from build123d import *

# Parameters (mm, degrees)
PAD_DEPTH       = 3
POCKET_DEPTH    = 2
SKETCH004_W     = 50
SKETCH004_H     = 84
SKETCH004_W_2   = 47.6
SKETCH004_H_2   = 81.6
POCKET001_DEPTH = 2
SKETCH005_R     = 3.5
SKETCH005_R_2   = 3
PAD001_DEPTH    = 6
SKETCH_R        = 1.8
POCKET002_DEPTH = 5


with BuildPart() as part:
    # Sketch002 → Pad (new body)
    with BuildSketch(Plane(origin=(0, 1, 0), x_dir=(-1, 0, 0), z_dir=(0, 1, 0))):
        Polygon((-44, -64), (2, -64), (2, 20), (-44, 20), (-48, 20), (-48, -64), align=None)
    extrude(amount=PAD_DEPTH)

    # Sketch003 → Pocket (cut)
    with BuildSketch(Plane(origin=(0, 1, 0), x_dir=(-1, 0, 0), z_dir=(0, 1, 0))):
        Polygon((-42, -62), (0, -62), (0, 18), (-42, 18), (-46, 18), (-46, -62), align=None)
    extrude(amount=POCKET_DEPTH, mode=Mode.SUBTRACT)

    # Sketch004 → Pocket001 (cut)
    with BuildSketch(Plane(origin=(0, 1, 0), x_dir=(-1, 0, 0), z_dir=(0, 1, 0))):
        with Locations((-23, -22)):
            Rectangle(SKETCH004_W, SKETCH004_H)
        with Locations((-23, -22)):
            Rectangle(SKETCH004_W_2, SKETCH004_H_2, mode=Mode.SUBTRACT)
    extrude(amount=POCKET001_DEPTH, mode=Mode.SUBTRACT)

    # Sketch005 (on Face4 of Pocket001) → Pad001 (join)
    with BuildSketch(Plane(origin=(0, 4, 0), x_dir=(-1, 0, 0), z_dir=(0, 1, 0))):
        with Locations((-33.499998, -54)):
            Circle(SKETCH005_R)
        with Locations((-8.499999, -53.999999)):
            Circle(SKETCH005_R)
        with Locations((-38.250001, -16.5)):
            Circle(SKETCH005_R_2)
        with Locations((-3.75, -16.5)):
            Circle(SKETCH005_R_2)
    extrude(amount=-PAD001_DEPTH)

    # Sketch (on Face30 of Pad001) → Pocket002 (cut)
    with BuildSketch(Plane(origin=(0, -2, 0), x_dir=(-1, 0, 0), z_dir=(0, -1, 0))):
        with Locations((-33.499998, 54)):
            Circle(SKETCH_R)
        with Locations((-8.499999, 53.999999)):
            Circle(SKETCH_R)
        with Locations((-38.250001, 16.5)):
            Circle(SKETCH_R)
        with Locations((-3.75, 16.5)):
            Circle(SKETCH_R)
    extrude(amount=-POCKET002_DEPTH, mode=Mode.SUBTRACT)


solid = part.part
Verification items for the finished model (mm, model axes). A direction names the side the tool comes from. Coordinates: 2 decimals unless noted, no trailing zeros. Write each loop counter-clockwise with the first axis right and the second up, starting at its lowest first coordinate (ties: lowest second). Pieces come first, ordered by that corner, then holes. Notation, with made-up numbers: M -20,46 L -14,46 A15 cw -14,61 Z; hole C 80.25,31 d9. An arc over 180 degrees is marked long. Use a Markdown table: item, result.
Q1. Draft check along Z on faces 6 (the face through (23, 2, -62.8)), 7 (the face through (46, 2, -21)), 8 (the face through (47, 3, -22)). Enter one of: +Z half, -Z half, draft (parallel to the pull), parting line (faces both ways), or undercut.
Reply:
| item | result |
|---|---|
| face 6 | -Z half |
| face 7 | undercut |
| face 8 | draft |
Q2. Sectioned sample at A-A, the plane y = -1.2. Record the boundary of the cut face in (x, z), plus the area to 3 significant figures.
Reply:
| item | result |
|---|---|
| outline | C 3.75,-16.5 d6; C 8.5,-54 d7; C 33.5,-54 d7; C 38.25,-16.5 d6; hole C 3.75,-16.5 d3.6; hole C 8.5,-54 d3.6; hole C 33.5,-54 d3.6; hole C 38.25,-16.5 d3.6 |
| area | 92.8 mm² |
Q3. Sectioned sample at C-C, the plane z = -23. Record the boundary of the cut face in (x, y), plus the area to 3 significant figures.
Reply:
| item | result |
|---|---|
| outline | M -2,3 L -0.8,3 L -0.8,1 L 0,1 L 0,3 L 46,3 L 46,1 L 46.8,1 L 46.8,3 L 48,3 L 48,4 L -2,4 Z |
| area | 53.2 mm² |
Q4. Thickness scan on line 1 (X direction, y = 1.3, z = 12.5); line 2 (X direction, y = -0.85, z = -55.5); line 3 (Z direction, x = 38.25, y = 0.25). Record the ranges inside material, lowest first.
Reply:
| item | result |
|---|---|
| line 1 | x = -0.8 to 0, 46 to 46.8 |
| line 2 | x = 5.34 to 7.51, 9.49 to 11.66, 30.34 to 32.51, 34.49 to 36.66 |
| line 3 | z = -19.5 to -18.3, -14.7 to -13.5 |
Q5. Sectioned sample at D-D, the plane x = 19. Record the boundary of the cut face in (y, z), plus the area to 3 significant figures.
Reply:
| item | result |
|---|---|
| outline | M 1,-62.8 L 3,-62.8 L 3,-64 L 4,-64 L 4,20 L 3,20 L 3,18.8 L 1,18.8 L 1,18 L 3,18 L 3,-62 L 1,-62 Z |
| area | 87.2 mm² |
Q6. Go/stop test with flat-tipped pins: P1, Ø0.6, axis at y = 2, z = -13, coming from the -X side; P2, Ø0.6, axis at x = 21.5, y = 2.5, coming from the -Z side; P3, Ø1.6, axis at x = 24, y = 2, coming from the +Z side. Record where each tip stops, or that it passes through.
Reply:
| item | result |
|---|---|
| P1 | stops at x = -0.8 |
| P2 | stops at z = -62.8 |
| P3 | stops at z = 18.8 |
Q7. Set-up check for faces 1 (the face through (23, 4, -21)), 2 (the face through (-0.8, 2, -23)), 3 (the face through (37, -2, -18)), 4 (the face through (34, 3, -54)), 5 (the face through (46.8, 2, -23)): record each of +Z, -Z, +X, -X, +Y, -Y from which the full face is reachable in a straight line by a thin tool's end or side.
Reply:
| item | result |
|---|---|
| face 1 | +Z, -Z, +X, -X, +Y |
| face 2 | +Z, -Z, -X, -Y |
| face 3 | +Z, -Z, +X, -X, -Y |
| face 4 | -Y |
| face 5 | +Z, -Z, +X, -Y |
Q8. Sectioned sample at B-B, the plane x = 8.5. Record the boundary of the cut face in (y, z), plus the area to 3 significant figures.
Reply:
| item | result |
|---|---|
| outline | M -2,-57.5 L 3,-57.5 L 3,-62 L 1,-62 L 1,-62.8 L 3,-62.8 L 3,-64 L 4,-64 L 4,20 L 3,20 L 3,18.8 L 1,18.8 L 1,18 L 3,18 L 3,-50.5 L -2,-50.5 L -2,-52.2 L 3,-52.2 L 3,-55.8 L -2,-55.8 Z |
| area | 104 mm² |
